Could you check a few things on this model? Use its own coordinates, in mm. A direction names the side the tool comes from. Give positions to 0.01 mm unless a question says otherwise; leave off trailing zeros. Loops run counter-clockwise (first coordinate to the right, second up) from the corner with the lowest first, then second, coordinate; pieces in that order, holes last. Notation, with made-up numbers: M 20.25,-14.5 L 25.25,-14.5 A19 cw 25.25,19.5 Z; hole C 52,34.25 d8. An arc over 180 degrees is marked long. Answer in a Markdown table with one row per item. Add a question column.
1. If we section it at B-B on z = 25: List the corners of the cut face in (x, y) for me.
2. If we section it at A-A on x = 37: List the corners of the cut face in (y, z) for me.
3. I need wall thicknesses on line 1 along X through (y, z) = (14, 25); line 2 along X through (y, z) = (38, 25); line 3 along X through (y, z) = (39, 40). Which ranges of each line are inside material? Lowest first, please. Write a range as from..to.
4. Which directions (+Z, -Z, +X, -X, +Y, -Y) give clear straight access to the entire face, cutting with the end or side of a thin tool? Please do faces 1 (the flat face through (-10, 43, 43)), 2 (the flat face through (-28, 30, 30)), 3 (the flat face through (28.5, 15, 19.1)).
5. If we section it at C-C on z = 43: List the corners of the cut face in (x, y) for me.
6. If we section it at D-D on y = 45.5: List the corners of the cut face in (x, z) for me, then the cut area to 3 significant figures.
7. Thinking about a two-plate mould opening in X: for faces 4 (the flat face through (20, 32, 25)), 5 (the cylindrical face through (0.51, 42.6, 10.01)), 6 (the flat face through (-50, 15, 25)), 7 (the flat face through (10, 43, 43)), which applies, released by +X, released by -X, zero draft, split by the parting line, or undercut?
8. I'm going to push flat-ended pins straight in: pin 1 Ø1 at (x, z) = (1.5, 33.5) entering from +Y; pin 2 Ø15 at (y, z) = (39, 40) entering from -X; pin 3 Ø3 at (x, z) = (-17.5, 31.5) entering from -Y; pin 4 Ø17.5 at (y, z) = (41, 19.5) entering from +X. Where does each tip first touch, or does it pass through?
```python
from build123d import *

# Parameters (mm, degrees)
RESSALTO_EXTRUS_O1_DEPTH = 50
ESBO_O2_R                = 10
ESBO_O2_R_2              = 10.000432036
CORTE_EXTRUS_O1_DEPTH    = 87.602540378
ESBO_O3_R                = 15
CORTE_EXTRUS_O2_DEPTH    = 15
CORTE_EXTRUS_O3_DEPTH    = 15


with BuildPart() as part:
    # Esboço1 → Ressalto-extrusão1 (new body)
    with BuildSketch(Plane.XY):
        Polygon((-50, 0), (50, 0), (50, 15), (20, 15), (20, 50), (-20, 50), (-20, 30), (-50, 30), align=None)
    extrude(amount=RESSALTO_EXTRUS_O1_DEPTH)

    # Esboço2 → Corte-extrusão1 (cut, through all)
    with BuildSketch(Plane(origin=(0, 50, 0), x_dir=(1, 0, 0), z_dir=(0, 1, 0))):
        with Locations(Location((-37, -25, 0), (0, 0, 270))):
            Circle(ESBO_O2_R)
        with Locations(Location((37, -25, 0), (0, 0, 270))):
            Circle(ESBO_O2_R_2)
    extrude(amount=-CORTE_EXTRUS_O1_DEPTH, mode=Mode.SUBTRACT)

    # Esboço3 → Corte-extrusão2 (cut)
    with BuildSketch(Plane(origin=(0, 50, 0), x_dir=(1, 0, 0), z_dir=(0, 1, 0))):
        with Locations(Location((0, -25, 0), (0, 0, 270))):
            Circle(ESBO_O3_R)
    extrude(amount=-CORTE_EXTRUS_O2_DEPTH, mode=Mode.SUBTRACT)

    # Esboço5 → Corte-extrusão3 (cut)
    with BuildSketch(Plane(origin=(0, 50, 0), x_dir=(1, 0, 0), z_dir=(0, 1, 0))):
        with BuildLine():
            Line((-10, -36.180339887), (-10, -50))
            Line((-10, -50), (10, -50))
            Line((10, -50), (10, -36.180339887))
            ThreePointArc((10, -36.180339887), (0, -40), (-10, -36.180339887))
        make_face()
    extrude(amount=-CORTE_EXTRUS_O3_DEPTH, mode=Mode.SUBTRACT)


solid = part.part
```
Results:
| question | item | result |
|---|---|---|
| 1 | outline | M -50,0 L -47,0 L -47,30 L -50,30 Z; M -27,0 L 27,0 L 27,15 L 20,15 L 20,50 L 15,50 L 15,35 L -15,35 L -15,50 L -20,50 L -20,30 L -27,30 Z; M 47,0 L 50,0 L 50,15 L 47,15 Z |
| 2 | outline | M 0,0 L 15,0 L 15,15 L 0,15 Z; M 0,35 L 15,35 L 15,50 L 0,50 Z |
| 3 | line 1 | -50..-47, -27..27, 47..50 |
| 3 | line 2 | -20..-15, 15..20 |
| 3 | line 3 | -20..-10, 10..20 |
| 4 | face 1 | +Z, +Y |
| 4 | face 2 | +Z, -Z, -X, +Y |
| 4 | face 3 | +Z, -Z, +X, +Y |
| 5 | outline | M -50,0 L 50,0 L 50,15 L 20,15 L 20,50 L 10,50 L 10,35 L -10,35 L -10,50 L -20,50 L -20,30 L -50,30 Z |
| 6 | outline | M -20,0 L 20,0 L 20,50 L 10,50 L 10,36.18 A15 cw long -10,36.18 L -10,50 L -20,50 Z |
| 6 | area | 1,070 mm2 |
| 7 | face 4 | released by +X |
| 7 | face 5 | undercut |
| 7 | face 6 | released by -X |
| 7 | face 7 | undercut |
| 8 | pin 1 | y = 35 |
| 8 | pin 2 | x = -20 |
| 8 | pin 3 | y = 0 |
| 8 | pin 4 | x = 20 |
